Autodesk Inventor part; units mm, degrees
ref_plane "YZ Plane" through (0, 0, 0) normal (1, 0, 0) x (0, 1, 0)
ref_plane "XZ Plane" through (0, 0, 0) normal (0, 1, 0) x (-1, 0, 0)
ref_plane "XY Plane" through (0, 0, 0) normal (0, 0, 1) x (1, 0, 0)
sketch "Sketch1" plane through (0, 0, 0) normal (0, 0, 1) x (1, 0, 0)
  line L0 (0, 0) -> (31.75, 0)
  arc A0 (0, 12.7) -> (31.75, 12.7) centre (15.875, 60.9558) ccw
  line L1 (0, 12.7) -> (0, 0)
  line L2 (31.75, 12.7) -> (31.75, 0)
  dimension "d0" = 50.8
  dimension "d1" = 31.75
  dimension "d2" = 12.7
extrude "Extrusion1" add sketch "Sketch1" along normal blind 31.75
sketch "Sketch2" plane through (0, 0, 0) normal (0, -1, 0) x (1, 0, 0)
  line L0 (31.75, 0) -> (31.75, 31.75)
  circle A0 centre (15.875, 15.875) radius 12.7
  line L1 (0, 0) -> (31.75, 0)
  line L2 (15.875, 15.875) -> (0, 15.875) construction
  line L3 (0, 0) -> (0, 31.75) construction
  line L4 (15.875, 15.875) -> (31.75, 15.875) construction
  line L5 (15.875, 15.875) -> (15.875, 31.75) construction
  line L6 (15.875, 15.875) -> (15.875, 0) construction
  line L7 (0, 31.75) -> (31.75, 31.75) construction
  dimension "d5" = 25.4
extrude "Extrusion2" cut sketch "Sketch2" against normal through all
fillet "Fillet1" radius 3.175 4 edges at (31.75, 6.35, 31.75) (0, 6.35, 31.75) (31.75, 6.35, 0) (0, 6.35, 0)
properties part number "CoilHolder" material "ABS Plastic"
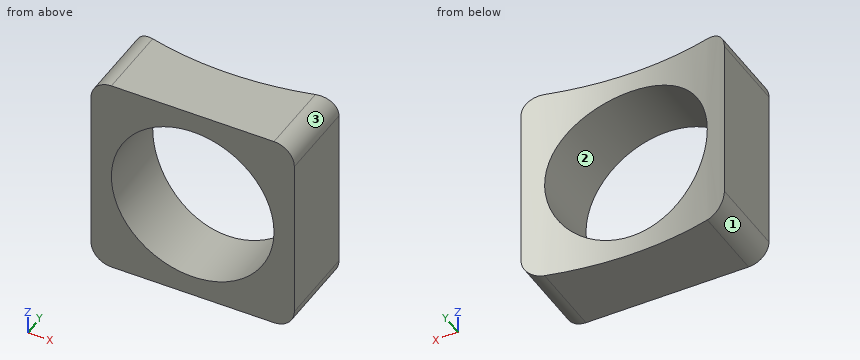
Could you check a few things on this model? Use its own coordinates, in mm. Face numbers are marked on the shaded views. Round coordinates to 2 decimals unless told otherwise and drop trailing zeros. Loops run counter-clockwise (first coordinate to the right, second up) from the corner with the lowest first, then second, coordinate; pieces in that order, holes last. Notation, with made-up numbers: (64, -22.75) - (112, -22.75) arc R22 cw to (112, 0.25) - close; hole circle Ø5 at (-17, 9.25). An arc over 180 degrees is marked (long way). Use CSV: the item, a comma, the result in double quotes.
Item 1: Will this pin go through, and if not, where does the flat tip stop? pin 1 (6 mm diameter, centred on x = 6, z = 5, fed in from +Y).
Here are the results:
pin 1,"stops at y = 11.81"
Item 2: If we section it at C-C on y = 10.75: List the corners of the cut face in (x, z) for me (3 decimals), then the cut area to 3 significant figures.
Here are the results:
outline,"(0, 3.175) arc R3.175 ccw to (3.175, 0) - (8.128, 0) - (8.128, 5.811) arc R12.7 cw to (8.128, 25.939) - (8.128, 31.75) - (3.175, 31.75) arc R3.175 ccw to (0, 28.575) - close; (23.622, 0) - (28.575, 0) arc R3.175 ccw to (31.75, 3.175) - (31.75, 28.575) arc R3.175 ccw to (28.575, 31.75) - (23.622, 31.75) - (23.622, 25.939) arc R12.7 cw to (23.622, 5.811) - close"
area,"368 mm²"
Item 3: I need wall thicknesses on L1, parallel to X at y = 7.25, z = 3; L2, parallel to Z at x = 8.5, y = 6.25; L3, parallel to Z at x = 13, y = 5.75. Which ranges of each line are inside material? Lowest first, please. Write a range as [from, to].
Here are the results:
L1,"x = [0, 31.75]"
L2,"z = [0, 5.54], [26.21, 31.75]"
L3,"z = [0, 3.5], [28.25, 31.75]"
Item 4: If we mould it in two halves opening along X, with no side actions, what happens to the marked faces 1, 2 and 3? For each: pulls with the +X half, pulls with the -X half, needs draft (parallel to the pull), parting line crosses it, or undercut.
Here are the results:
face 1,"pulls with the -X half"
face 2,"undercut"
face 3,"pulls with the +X half"
Item 5: If we section it at A-A on x = 14.5: List the corners of the cut face in (y, z) for me, then the cut area to 3 significant figures.
Here are the results:
outline,"(0, 0) - (10.17, 0) - (10.17, 3.25) - (0, 3.25) - close; (0, 28.5) - (10.17, 28.5) - (10.17, 31.75) - (0, 31.75) - close"
area,"66.1 mm²"
Item 6: If we section it at B-B on z = 18: List the corners of the cut face in (x, y) for me (3 decimals), then the cut area to 3 significant figures.
Here are the results:
outline,"(0, 0) - (3.354, 0) - (3.354, 11.723) arc R50.8 cw to (0, 12.7) - close; (28.396, 0) - (31.75, 0) - (31.75, 12.7) arc R50.8 cw to (28.396, 11.723) - close"
area,"81.8 mm²"
